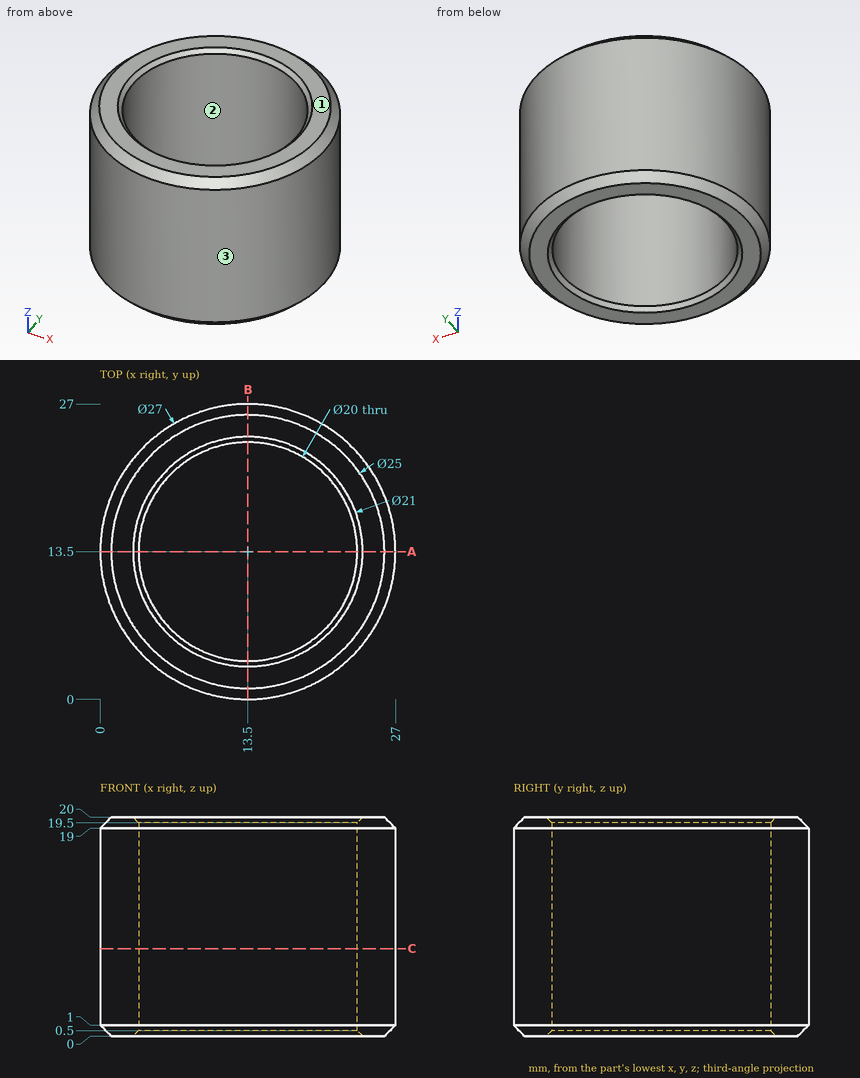
Design review of the part shown in the three views and the two pictorial views. Dimensions are in mm from the part's minimum x, y and z. Round coordinates to 2 decimals unless told otherwise and drop trailing zeros. Loops run counter-clockwise (first coordinate to the right, second up) from the corner with the lowest first, then second, coordinate; pieces in that order, holes last.
1) Clearance check with flat-ended pins moving along their axes: P1, Ø5, axis at x = 10, z = 7.5, coming from the -Y side; P2, Ø3, axis at x = 11, z = 14, coming from the +Y side; P3, Ø1, axis at y = 11, z = 17.5, coming from the -X side. State where each tip first meets the part, or that it passes through.
Values follow:
P1: stops at y = 0.04
P2: stops at y = 26.96
P3: stops at x = 0.15
2) Consider section C-C on z = 8. State the section outline as (x, y) points, then the cut area to 3 significant figures.
Values follow:
outline: circle Ø27 at (13.5, 13.5); hole circle Ø20 at (13.5, 13.5)
area: 258 mm2
3) The part is to be moulded in two halves that separate along Y. For the marked faces 1, 2 and 3, say which applies: pulls with the +Y half, pulls with the -Y half, needs draft (parallel to the pull), parting line crosses it, or undercut.
Values follow:
face 1: needs draft
face 2: undercut
face 3: parting line crosses it
4) Consider section A-A on y = 13.5. State the section outline as (x, z) points.
Values follow:
outline: (0, 1) - (1, 0) - (3, 0) - (3.5, 0.5) - (3.5, 19.5) - (3, 20) - (1, 20) - (0, 19) - close; (23.5, 0.5) - (24, 0) - (26, 0) - (27, 1) - (27, 19) - (26, 20) - (24, 20) - (23.5, 19.5) - close
5) Wall thickness on line 1 along Y through (x, z) = (13.5, 15.5); line 2 along X through (y, z) = (19, 5.75); line 3 along Y through (x, z) = (12, 9.5): over which ranges is each line inside the solid? List them lowest first.
Values follow:
line 1: y = 0 to 3.5, 23.5 to 27
line 2: x = 1.17 to 5.15, 21.85 to 25.83
line 3: y = 0.08 to 3.61, 23.39 to 26.92
